```python
from build123d import *

# Parameters (mm, degrees)
BOSS_EXTRUDE1_DEPTH = 25.4
SKETCH2_W           = 50.8
SKETCH2_H           = 127
BOSS_EXTRUDE2_DEPTH = 6.35
SKETCH3_R           = 4.7625
CUT_EXTRUDE1_DEPTH  = 86.194189943
BOSS_EXTRUDE3_DEPTH = 6.35


with BuildPart() as part:
    # Sketch1 → Boss-Extrude1 (new body)
    with BuildSketch(Plane(origin=(0, 0, 0), x_dir=(1, 0, 0), z_dir=(0, 1, 0))):
        with BuildLine():
            Line((0, 33.02), (0, 63.5))
            Line((0, 63.5), (-50.8, 63.5))
            Line((-50.8, 63.5), (-50.8, -63.5))
            Line((-50.8, -63.5), (0, -63.5))
            Line((0, -63.5), (0, -33.02))
            ThreePointArc((0, -33.02), (-33.02, 0), (0, 33.02))
        make_face()
    extrude(amount=BOSS_EXTRUDE1_DEPTH)

    # Sketch2 → Boss-Extrude2 (add)
    with BuildSketch(Plane.XZ):
        with Locations((-25.4, 0)):
            Rectangle(SKETCH2_W, SKETCH2_H)
    extrude(amount=BOSS_EXTRUDE2_DEPTH)

    # Sketch3 → Cut-Extrude1 (cut, through all)
    with BuildSketch(Plane(origin=(0, 0, 0), x_dir=(0, 0, -1), z_dir=(1, 0, 0))):
        with Locations((-48.26, 12.7)):
            Circle(SKETCH3_R)
        with Locations(Location((48.26, 12.7, 0), (0, 0, 180))):
            Circle(SKETCH3_R)
    extrude(amount=-CUT_EXTRUDE1_DEPTH, mode=Mode.SUBTRACT)

    # Sketch4 → Boss-Extrude3 (add)
    with BuildSketch(Plane(origin=(0, 0, 0), x_dir=(1, 0, 0), z_dir=(0, 1, 0))):
        Polygon((-3.592850725, 6.223), (-7.18570145, 0), (-3.592850725, -6.223), (0, -6.223), (0, 6.223), align=None)
    extrude(amount=BOSS_EXTRUDE3_DEPTH)


solid = part.part
```
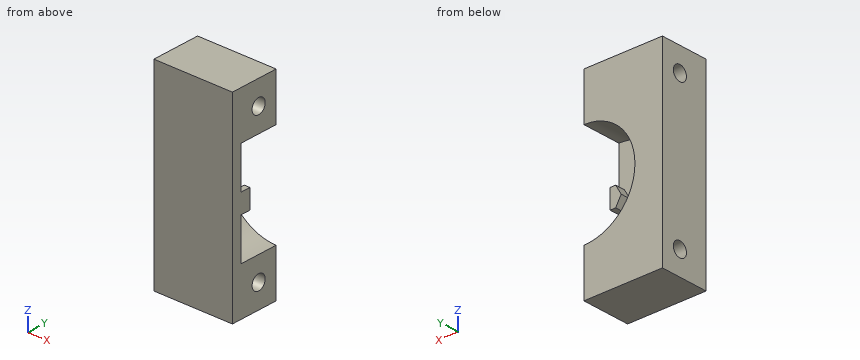
Could you check a few things on this model? Use its own coordinates, in mm. Round coordinates to 2 decimals unless told otherwise and drop trailing zeros. Write each loop counter-clockwise with the first axis right and the second up, starting at its lowest first coordinate (ties: lowest second). Pieces come first, ordered by that corner, then holes.
(1) Suppose I cut it at A-A on y = 12.7. Write out the boundary of the cut face in (x, z), and give its area (3 significant figures).
Findings below:
outline: (-50.8, -63.5) - (0, -63.5) - (0, -53.02) - (-50.8, -53.02) - close; (-50.8, -43.5) - (0, -43.5) - (0, -33.02) arc R33.02 cw to (0, 33.02) - (0, 43.5) - (-50.8, 43.5) - close; (-50.8, 53.02) - (0, 53.02) - (0, 63.5) - (-50.8, 63.5) - close
area: 3,770 mm2
(2) For pin 1 (16.5 mm diameter, centred on x = -14.5, z = 6.5, fed in from +Y); pin 2 (2 mm diameter, centred on x = -3, z = -1, fed in from +Y); pin 3 (10 mm diameter, centred on y = 8, z = 3, fed in from +X), each with a flat end and sliding along its axis, tell me the tip position at first contact or that it passes through.
Findings below:
pin 1: stops at y = 0
pin 2: stops at y = 6.35
pin 3: stops at x = 0
(3) Suppose I cut it at B-B on z = -48.26. Write out the boundary of the cut face in (x, y), and give its area (3 significant figures).
Findings below:
outline: (-50.8, -6.35) - (0, -6.35) - (0, 7.94) - (-50.8, 7.94) - close; (-50.8, 17.46) - (0, 17.46) - (0, 25.4) - (-50.8, 25.4) - close
area: 1,130 mm2
(4) Suppose I cut it at C-C on y = 2.5. Write out the boundary of the cut face in (x, z).
Findings below:
outline: (-50.8, -63.5) - (0, -63.5) - (0, -33.02) arc R33.02 cw to (0, 33.02) - (0, 63.5) - (-50.8, 63.5) - close; (-7.19, 0) - (-3.59, -6.22) - (0, -6.22) - (0, 6.22) - (-3.59, 6.22) - close
(5) Suppose I cut it at D-D on x = -17. State how many separate pieces and enclosed holes the cut face has, and give its area (3 significant figures).
Findings below:
separate pieces: 1
enclosed holes: 2
area: 2,450 mm2
(6) If I drill on probe 1 along Y at (x, z) = (-36, -48); probe 2 along Z at (x, y) = (-18, 14); probe 3 along Y at (x, z) = (-20.5, 21), over which ranges is the centre line in solid material (lowest first)?
Findings below:
probe 1: y = -6.35 to 7.94, 17.46 to 25.4
probe 2: z = -63.5 to -52.84, -43.68 to -27.68, 27.68 to 43.68, 52.84 to 63.5
probe 3: y = -6.35 to 0
